For this review, take the finished solid that the model builds, in its own axes (mm). Face numbers are marked on the shaded views. A direction names the side the tool comes from. Coordinates: 2 decimals unless noted, no trailing zeros. Loops run counter-clockwise (first coordinate to the right, second up) from the corner with the lowest first, then second, coordinate; pieces in that order, holes last. Notation, with made-up numbers: M -16.75,71.5 L -1.75,71.5 A23 ccw -1.75,80.5 Z; hole C 14.5,80.25 d8. An arc over 180 degrees is marked long. Write each question's results on one line, items separated by ' | '. Start each with the question number.
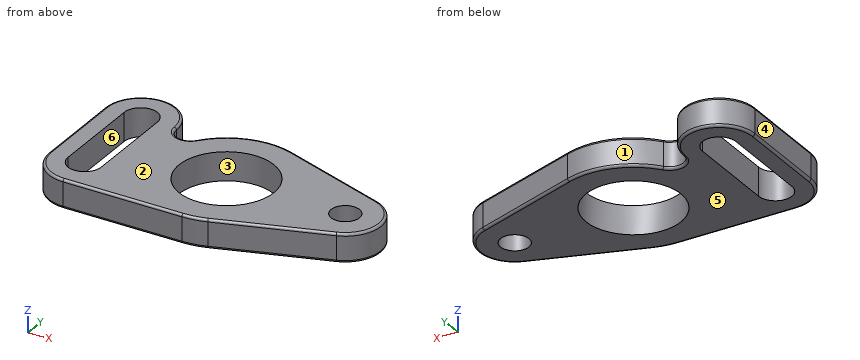
```python
from build123d import *

# Parameters (mm, degrees)
SKETCH_R    = 20
SKETCH_R_2  = 6
PAD_DEPTH   = 12
FILLET_R    = 1
FILLET001_R = 1


with BuildPart() as part:
    # Sketch → Pad (new body)
    with BuildSketch(Plane.XY):
        with BuildLine():
            ThreePointArc((0, -31), (5.026517, -30.589772), (9.92, -29.369944))
            Line((9.92, -29.369944), (54.8, -14.211263))
            ThreePointArc((54.8, -14.211263), (65, 0), (54.8, 14.211263))
            Line((54.8, 14.211263), (9.919999, 29.369944))
            ThreePointArc((9.919999, 29.369944), (-8.790322, 29.727601), (-24.297307, 19.252036))
            ThreePointArc((-35.000008, 22.984455), (-30.975734, 17.312857), (-24.297307, 19.252036))
            ThreePointArc((-35.000008, 22.984455), (-49.992227, 37.999998), (-65, 23))
            Line((-65, 23), (-65, -16))
            ThreePointArc((-65, -16), (-60.606602, -26.606602), (-50, -31))
            Line((-50, -31), (0, -31))
        make_face()
        Circle(SKETCH_R, mode=Mode.SUBTRACT)
        with Locations((50, 0)):
            Circle(SKETCH_R_2, mode=Mode.SUBTRACT)
        with BuildLine():
            ThreePointArc((-57, -16), (-50.000013, -23), (-43, -16.000027))
            Line((-43, 23), (-43, -16.000027))
            ThreePointArc((-43, 23), (-50, 30), (-57, 23))
            Line((-57, -16), (-57, 23))
        make_face(mode=Mode.SUBTRACT)
    extrude(amount=PAD_DEPTH)

    # Fillet
    fillet_edges = [part.edges().sort_by_distance(p)[0] for p in [
        (32.36, -21.790603, 12),
        (5.026517, -30.589772, 12),
        (-25, -31, 12),
        (-60.606602, -26.606602, 12),
        (-65, 3.5, 12),
        (-49.992227, 37.999998, 12),
        (-30.975734, 17.312857, 12),
        (-8.790322, 29.727601, 12),
        (32.36, 21.790604, 12),
        (65, 0, 12),
    ]]
    fillet(fillet_edges, radius=FILLET_R)

    # Fillet001
    fillet001_edges = [part.edges().sort_by_distance(p)[0] for p in [
        (5.026517, -30.589772, 0),
        (-25, -31, 0),
        (-60.606602, -26.606602, 0),
        (-65, 3.5, 0),
        (-49.992227, 37.999998, 0),
        (-30.975734, 17.312857, 0),
        (-8.790322, 29.727601, 0),
        (32.36, 21.790604, 0),
        (65, 0, 0),
        (32.36, -21.790603, 0),
    ]]
    fillet(fillet001_edges, radius=FILLET001_R)


solid = part.part
```
Q1. Take a section at B-B, the plane y = -17.5. Give the number of separate pieces and of enclosed holes in the cut face, then the cut area to 3 significant figures.
Q2. Insertion check: P1, Ø2, axis at x = 37.5, y = -4, coming from the -Z side; P2, Ø6, axis at y = 8, z = 5.5, coming from the +X side; P3, Ø3, axis at x = -22, z = 10.5, coming from the +Y side; P4, Ø1.5, axis at x = -13.5, y = 28.5, coming from the +Z side. Each pin has a flat end and moves straight along its axis. Give the tip position at first contact, or say it passes through.
Q3. To check wall thickness, follow line 1 along Y through (x, z) = (0, 2.5); line 2 along X through (y, z) = (9, 7.75); line 3 along Y through (x, z) = (50, 8.5). State the ranges of each line that lie inside material, in increasing order.
Q4. Take a section at A-A, the plane z = 2.75. Give the boundary of the cut face in (x, y), then the cut area to 3 significant figures.
Q5. The part is to be moulded in two halves that separate along X. For the marked faces 1, 2, 3 and 4, say which applies: pulls with the +X half, pulls with the -X half, needs draft (parallel to the pull), parting line crosses it, or undercut.
Q6. For the marked faces 5 and 6, list the 3-axis set-ups (+Z, -Z, +X, -X, +Y, -Y) from which the entire face can be reached by the end or side of a thin tool; tool diameter is ignored.
Results:
1) separate pieces: 3 | enclosed holes: 0 | area: 922 mm^2
2) P1: z = 0 | P2: x = 64.14 | P3: y = 23.25 | P4: z = 11.62
3) line 1: -31 to -20, 20 to 31 | line 2: -65 to -57, -43 to -17.86, 17.86 to 62 | line 3: -15.83 to -6, 6 to 15.83
4) outline: M -65,-16 A15 ccw -50,-31 L 0,-31 A31 ccw 9.92,-29.37 L 54.8,-14.21 A15 ccw 54.8,14.21 L 9.92,29.37 A31 ccw -24.3,19.25 A6 cw -35,22.98 A15 ccw -65,23 Z; hole M -57,-16 A7 ccw -43,-16 L -43,23 A7 ccw -57,23 Z; hole C 0,0 d40; hole C 50,0 d12 | area: 4,570 mm^2
5) face 1: undercut | face 2: needs draft | face 3: undercut | face 4: pulls with the -X half
6) face 5: -Z, +X, -X, +Y, -Y | face 6: +Z, -Z
